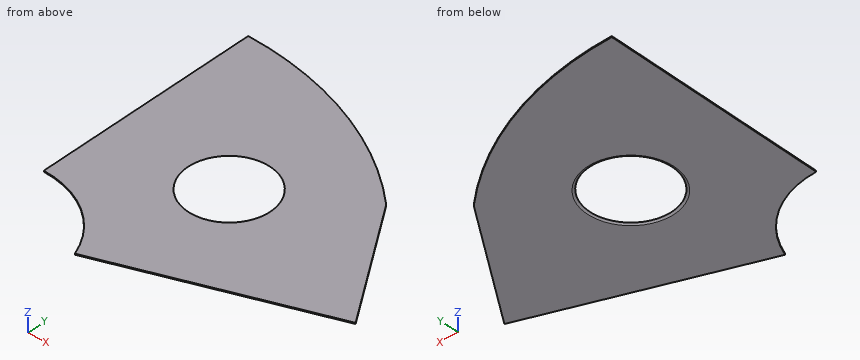
Solid Edge part; units mm, degrees
sketch "Sketch1" plane through (0, 0, 0) normal (0, 0, 1) x (1, 0, 0)
  line L0 (0.4572, 558.7998) -> (0.4572, 1930.3999)
  arc A0 (1107.232, 1581.2911) -> (0.4572, 1930.3999) centre (0, 0) ccw
  arc A1 (1316.5296, 1411.8052) -> (1107.232, 1581.2911) centre (0, 0) ccw
  line L1 (1316.5296, 1411.8052) -> (1813.7231, 660.6278)
  line L2 (524.9437, 191.5504) -> (1813.7231, 660.6278)
  arc A2 (524.9437, 191.5504) -> (0.4572, 558.7998) centre (0, 0) ccw
extrude "Protrusion1" add sketch "Sketch1" against normal blind 6.35
sketch "Sketch2" plane through (713.8732, 1019.5166, 0) normal (0.8636, -0.5042, 0) x (0.5042, 0.8636, 0)
  arc A0 (0, 50.8) -> (647.7, -596.9) centre (0, -596.9) cw
  line L0 (647.7, -596.9) -> (0, -596.9)
  line L1 (0, -596.9) -> (0, 50.8)
revolve "RevolvedCutout1" cut sketch "Sketch2" angle 360 about axis through (713.8732, 1019.5166, 0) along (0, 0, -1)
Geometry: final body of the model. Coordinates: model frame, mm. Give positions to 0.01 mm unless a question says otherwise; leave off trailing zeros. Loops run counter-clockwise (first coordinate to the right, second up) from the corner with the lowest first, then second, coordinate; pieces in that order, holes last. Notation, with made-up numbers: (-8.75, 16) - (21.25, 16) arc R25 ccw to (21.25, 49) - close; hole circle Ø6 at (-35, -23). An arc over 180 degrees is marked (long way). Answer as CSV lines item,"result". Start each with the question number.
(1) Pin query (flat end, axial travel): P1, Ø3, axis at x = 1091.5, z = -1, coming from the -Y side; P2, Ø12, axis at x = 1141, y = 451.5, coming from the +Z side. Return the tip coordinate at first contact, or that it passes through.
(2) Section query B-B (y = 1211.5). Output: boundary loops of the cut face in (x, z), and give its area (3 significant figures).
(3) Section query A-A (x = 714.5). Output: boundary loops of the cut face in (y, z).
(4) Section query D-D (y = 1652). Output: boundary loops of the cut face in (x, z), and give its area (3 significant figures).
(5) Ray query, line 1 along X through (y, z) = (929.5, -5.5); line 2 along X through (y, z) = (673, -2.5); line 3 along Y through (x, z) = (255, -3.75). Return the intervals inside material, ascending. Write a range as [from, to].
(6) Section query C-C (z = -4.75). Output: boundary loops of the cut face in (x, y).
Worked answers:
1,P1,"stops at y = 397.21"
1,P2,"stops at z = 0"
2,outline,"(0.46, -6.35) - (529.73, -6.35) arc R618.59 cw to (551.49, 0) - (0.46, 0) - close; (876.26, 0) arc R618.59 cw to (898.02, -6.35) - (1449.11, -6.35) - (1449.11, 0) - close"
2,area,"7,000 mm^2"
3,outline,"(260.54, -6.35) - (753.5, -6.35) arc R647.7 cw to (768.07, 0) - (260.54, 0) - close; (1270.96, 0) arc R647.7 cw to (1285.53, -6.35) - (1793.3, -6.35) - (1793.3, 0) - close"
4,outline,"(0.46, -6.35) - (998.67, -6.35) - (998.67, 0) - (0.46, 0) - close"
4,area,"6,340 mm^2"
5,line 1,"x = [0.46, 465.56], [962.18, 1635.76]"
5,line 2,"x = [0.46, 1805.53]"
5,line 3,"y = [497.22, 1913.48]"
6,outline,"(0.46, 558.8) arc R558.8 cw to (524.94, 191.55) - (1813.72, 660.63) - (1316.53, 1411.81) arc R1930.4 ccw to (0.46, 1930.4) - close; hole circle Ø524.88 at (713.87, 1019.52)"
